```python
from build123d import *

# Parameters (mm, degrees)
ESQUISSE1_W        = 165
ESQUISSE1_H        = 165
ESQUISSE1_R        = 2
ESQUISSE1_R_2      = 10
BOSS_EXTRU_1_DEPTH = 5
BOSS_EXTRU_2_DEPTH = 5


with BuildPart() as part:
    # Esquisse1 → Boss.-Extru.1 (new body)
    with BuildSketch(Plane.XY):
        Rectangle(ESQUISSE1_W, ESQUISSE1_H)
        with Locations((-76.5, 76.5)):
            Circle(ESQUISSE1_R, mode=Mode.SUBTRACT)
        with Locations((-76.5, 0)):
            Circle(ESQUISSE1_R, mode=Mode.SUBTRACT)
        with Locations((-76.5, -76.5)):
            Circle(ESQUISSE1_R, mode=Mode.SUBTRACT)
        with Locations((76.5, -76.5)):
            Circle(ESQUISSE1_R, mode=Mode.SUBTRACT)
        with Locations((76.5, 0)):
            Circle(ESQUISSE1_R, mode=Mode.SUBTRACT)
        with Locations((76.5, 76.5)):
            Circle(ESQUISSE1_R, mode=Mode.SUBTRACT)
        Circle(ESQUISSE1_R, mode=Mode.SUBTRACT)
        with Locations((42.41686608, 42.443425371)):
            Circle(ESQUISSE1_R_2, mode=Mode.SUBTRACT)
    extrude(amount=BOSS_EXTRU_1_DEPTH)

    # Esquisse2 → Boss.-Extru.2 (add)
    with BuildSketch(Plane(origin=(0, 0, 0), x_dir=(-1, 0, 0), z_dir=(0, 0, -1))):
        with BuildLine():
            Line((4, 77.5), (4, 6.34428877))
            ThreePointArc((4, 6.34428877), (3.032395143, 6.859634079), (2, 7.228416147))
            Line((2, 7.228416147), (2, 12.228416147))
            Line((2, 12.228416147), (-2, 12.228416147))
            Line((-2, 12.228416147), (-2, 7.228416147))
            ThreePointArc((-2, 7.228416147), (-3.032395143, 6.859634079), (-4, 6.34428877))
            Line((-4, 6.34428877), (-4, 77.143871387))
            Line((-4, 77.143871387), (-2, 77.143871387))
            Line((-2, 77.143871387), (-2, 72.5))
            Line((-2, 72.5), (2, 72.5))
            Line((2, 72.5), (2, 77.491359298))
            Line((2, 77.491359298), (4, 77.5))
        make_face()
    extrude(amount=BOSS_EXTRU_2_DEPTH)


solid = part.part
```
Here's how the part is built. I have some questions about the finished solid (model axes, mm). A direction names the side the tool comes from. Give positions to 0.01 mm unless a question says otherwise; leave off trailing zeros. Loops run counter-clockwise (first coordinate to the right, second up) from the corner with the lowest first, then second, coordinate; pieces in that order, holes last. Notation, with made-up numbers: (-6, 56.5) -> (15, 56.5) arc R11 cw to (15, 75.5) -> close; hole circle Ø11 at (68, 29). An arc over 180 degrees is marked (long way). Use one line per item in the form item = value. Start each with the question number.
1) Imagine slicing it at C-C (x = -76.5). Please give me the cut outline in (y, z).
2) Imagine slicing it at A-A (x = 0). Please give me the cut outline in (y, z), then the cut area to 3 significant figures.
3) Please list where these lines run through material, in increasing order: line 1 along Y through (x, z) = (76.5, 1.05); line 2 along Z through (x, y) = (-73, 20); line 3 along X through (y, z) = (48, -2).
4) Which directions (+Z, -Z, +X, -X, +Y, -Y) give clear straight access to the entire face, cutting with the end or side of a thin tool? Please do faces 1 (the face through (-1, 82.5, 2)), 2 (the face through (4, 41, -2)), 3 (the face through (2, 10, -2)), 4 (the face through (-4, 42, -2)), 5 (the face through (2, 75, -2)).
5) For P1, Ø3, axis at x = 23.5, z = -2.5, coming from the +Y side; P2, Ø1.5, axis at x = 53.5, y = -0.5, coming from the -Z side; P3, Ø1.5, axis at y = 8.5, z = -3, coming from the -X side; P4, Ø1.2, axis at x = -1, z = -2, coming from the +Y side, each with a flat end and sliding along its axis, tell me the tip position at first contact or that it passes through.
6) Imagine slicing it at D-D (y = 16.5). Please give me the cut outline in (x, z).
7) Imagine slicing it at B-B (y = -76.5). Please give me the cut outline in (x, z).
8) Thinking about a two-plate mould opening in Y: for faces 6 (the face through (0, 12.228, -2)), 7 (the face through (-82.5, -1, 2)), 8 (the face through (78.408, 0.601, 2.465)), which applies, +Y half, -Y half, draft (parallel to the pull), parting line (faces both ways), or undercut?
Check values:
q1.outline = (-82.5, 0) -> (-78.5, 0) -> (-78.5, 5) -> (-82.5, 5) -> close; (-74.5, 0) -> (-2, 0) -> (-2, 5) -> (-74.5, 5) -> close; (2, 0) -> (74.5, 0) -> (74.5, 5) -> (2, 5) -> close; (78.5, 0) -> (82.5, 0) -> (82.5, 5) -> (78.5, 5) -> close
q2.outline = (-82.5, 0) -> (-2, 0) -> (-2, 5) -> (-82.5, 5) -> close; (2, 0) -> (12.23, 0) -> (12.23, -5) -> (72.5, -5) -> (72.5, 0) -> (82.5, 0) -> (82.5, 5) -> (2, 5) -> close
q2.area = 1,110 mm^2
q3.line_1 = -82.5 to -78.5, -74.5 to -2, 2 to 74.5, 78.5 to 82.5
q3.line_2 = 0 to 5
q3.line_3 = -4 to 4
q4.face_1 = +Z, -Z, +X, -X, +Y
q4.face_2 = -Z, +X, +Y, -Y
q4.face_3 = -Z, -Y
q4.face_4 = -Z, -X, +Y, -Y
q4.face_5 = -Z, +Y
q5.P1 = through
q5.P2 = 0
q5.P3 = -4
q5.P4 = 72.5
q6.outline = (-82.5, 0) -> (-4, 0) -> (-4, -5) -> (4, -5) -> (4, 0) -> (82.5, 0) -> (82.5, 5) -> (-82.5, 5) -> close
q7.outline = (-82.5, 0) -> (-78.5, 0) -> (-78.5, 5) -> (-82.5, 5) -> close; (-74.5, 0) -> (74.5, 0) -> (74.5, 5) -> (-74.5, 5) -> close; (78.5, 0) -> (82.5, 0) -> (82.5, 5) -> (78.5, 5) -> close
q8.face_6 = -Y half
q8.face_7 = draft
q8.face_8 = undercut
